from build123d import *

# Parameters (mm, degrees)
SKETCH_1_R          = 2.5
EXTRUDE_1_DEPTH     = 2.5
EXTRUDE_2_DEPTH     = 19
CUT_EXTRUDE_1_DEPTH = 19
SKETCH_4_R          = 2.5
CUT_EXTRUDE_2_DEPTH = 19


with BuildPart() as part:
    # 草图1 → 凸台-拉伸1 (new body)
    with BuildSketch(Plane(origin=(0, 0, 0), x_dir=(1, 0, 0), z_dir=(0, 1, 0))):
        with BuildLine():
            Line((23, -9.5), (-32.5, -9.5))
            Line((-32.5, -9.5), (-32.5, 9.5))
            Line((-32.5, 9.5), (23, 9.5))
            ThreePointArc((23, 9.5), (32.5, 0), (23, -9.5))
        make_face()
        with Locations((-15, 0)):
            Circle(SKETCH_1_R, mode=Mode.SUBTRACT)
        with Locations((17, 0)):
            Circle(SKETCH_1_R, mode=Mode.SUBTRACT)
    extrude(amount=EXTRUDE_1_DEPTH)

    # 草图2 → 凸台-拉伸2 (add)
    with BuildSketch(Plane.XY.offset(9.5)):
        Polygon((-35, 2.5), (-32.5, 0), (-32.5, 2.5), (-32.5, 67.5), (-35, 67.5), align=None)
    extrude(amount=-EXTRUDE_2_DEPTH)

    # 草图3 → 切除-拉伸1 (cut)
    with BuildSketch(Plane(origin=(-32.5, 0, 0), x_dir=(0, 0, -1), z_dir=(1, 0, 0))):
        with BuildLine():
            Line((9.5, 67.5), (0, 67.5))
            ThreePointArc((0, 67.5), (6.717514421, 64.717514421), (9.5, 58))
            Line((9.5, 58), (9.5, 67.5))
        make_face()
        with BuildLine():
            Line((0, 67.5), (-9.5, 67.5))
            Line((-9.5, 67.5), (-9.5, 58))
            ThreePointArc((-9.5, 58), (-6.717514421, 64.717514421), (0, 67.5))
        make_face()
    extrude(amount=-CUT_EXTRUDE_1_DEPTH, mode=Mode.SUBTRACT)

    # 草图4 → 切除-拉伸2 (cut)
    with BuildSketch(Plane(origin=(-32.5, 0, 0), x_dir=(0, 0, -1), z_dir=(1, 0, 0))):
        with Locations((0, 52)):
            Circle(SKETCH_4_R)
        with Locations((0, 20)):
            Circle(SKETCH_4_R)
    extrude(amount=-CUT_EXTRUDE_2_DEPTH, mode=Mode.SUBTRACT)


solid = part.part
Verification items for the finished model (mm, model axes). A direction names the side the tool comes from. Give positions to 0.01 mm unless a question says otherwise; leave off trailing zeros. Loops run counter-clockwise (first coordinate to the right, second up) from the corner with the lowest first, then second, coordinate; pieces in that order, holes last.
1) Draft check along Z on faces 3 (the flat face through (-33.8, 1.3, 0.1)), 4 (the flat face through (-34, 16, -9.5)), 5 (the cylindrical face through (-17.5, 1.2, -0.1)). Enter one of: pulls with the +Z half, pulls with the -Z half, needs draft (parallel to the pull), parting line crosses it, or undercut.
2) Set-up check for faces 1 (the flat face through (-32.5, 35, 0)), 2 (the cylindrical face through (-33.73, 22.48, 0.33)): record each of +Z, -Z, +X, -X, +Y, -Y from which the full face is reachable in a straight line by a thin tool's end or side.
3) Sectioned sample at A-A, the plane x = 17. Enter the section's corners in (y, z).
4) Sectioned sample at B-B, the plane y = 52. Enter the section's corners in (x, z), then the cut area to 3 significant figures.
5) Sectioned sample at C-C, the plane z = -7.5. Enter the section's corners in (x, y).
6) Depth check by flat-ended pin: pin 1 Ø6.5 at (y, z) = (20, 0) entering from +X; pin 2 Ø3 at (x, z) = (-16.5, 1.5) entering from +Y; pin 3 Ø4.5 at (x, z) = (17, 0) entering from +Y. Enter the tip coordinate at first touch or a pass-through.
7) Sectioned sample at D-D, the plane y = 33. Enter the section's corners in (x, z).
8) Thickness scan on line 1 along X through (y, z) = (1.3, 0); line 2 along X through (y, z) = (1.5, 0); line 3 along Y through (x, z) = (-34.5, 0). Record the ranges inside material, lowest first.
Answers:
1. face 3: needs draft
1. face 4: pulls with the -Z half
1. face 5: undercut
2. face 1: +Z, -Z, +X, +Y
2. face 2: +X, -X
3. outline: (0, -9.5) - (2.5, -9.5) - (2.5, -2.5) - (0, -2.5) - close; (0, 2.5) - (2.5, 2.5) - (2.5, 9.5) - (0, 9.5) - close
4. outline: (-35, -9.5) - (-32.5, -9.5) - (-32.5, -2.5) - (-35, -2.5) - close; (-35, 2.5) - (-32.5, 2.5) - (-32.5, 9.5) - (-35, 9.5) - close
4. area: 35.0 mm2
5. outline: (-35, 2.5) - (-32.5, 0) - (28.83, 0) - (28.83, 2.5) - (-32.5, 2.5) - (-32.5, 63.83) - (-35, 63.83) - close
6. pin 1: stops at x = -32.5
6. pin 2: stops at y = 2.5
6. pin 3: passes through
7. outline: (-35, -9.5) - (-32.5, -9.5) - (-32.5, 9.5) - (-35, 9.5) - close
8. line 1: x = -33.8 to -17.5, -12.5 to 14.5, 19.5 to 32.5
8. line 2: x = -34 to -17.5, -12.5 to 14.5, 19.5 to 32.5
8. line 3: y = 2 to 17.5, 22.5 to 49.5, 54.5 to 67.5
